```python
from build123d import *

# Parameters (mm, degrees)
SKETCH_1_W          = 5
SKETCH_1_H          = 20
SKETCH_1_H_2        = 5
SKETCH_1_W_2        = 20
EXTRUDE_1_DEPTH     = 20
CUT_EXTRUDE_1_REACH = 36.641
SKETCH_2_R          = 1.5
CUT_EXTRUDE_2_REACH = 39.749
SKETCH_3_R          = 1.5


with BuildPart() as part:
    # 草图1 → 凸台-拉伸1 (new body)
    with BuildSketch(Plane.XY):
        with Locations((2.5, -10)):
            Rectangle(SKETCH_1_W, SKETCH_1_H)
        with Locations((2.5, -22.5)):
            Rectangle(SKETCH_1_W, SKETCH_1_H_2)
        with Locations((-10, -22.5)):
            Rectangle(SKETCH_1_W_2, SKETCH_1_H_2)
    extrude(amount=EXTRUDE_1_DEPTH)

    # 草图2 → 切除-拉伸1 (cut, up to next)
    with BuildSketch(Plane(origin=(0, -20, 0), x_dir=(1, 0, 0), z_dir=(0, 1, 0)), mode=Mode.PRIVATE) as cut_extrude_1_sk1:
        with Locations(Location((-10, -10, 0), (0, 0, 180))):
            Circle(SKETCH_2_R)
    cut_extrude_1_tool1 = extrude(cut_extrude_1_sk1.sketch, amount=-CUT_EXTRUDE_1_REACH, mode=Mode.PRIVATE) & part.part
    add(cut_extrude_1_tool1.solids().sort_by_distance((-10, -20, 10))[0], mode=Mode.SUBTRACT)

    # 草图3 → 切除-拉伸2 (cut, up to next)
    with BuildSketch(Plane.ZY, mode=Mode.PRIVATE) as cut_extrude_2_sk1:
        with Locations(Location((10, -10, 0), (0, 0, 270))):
            Circle(SKETCH_3_R)
    cut_extrude_2_tool1 = extrude(cut_extrude_2_sk1.sketch, amount=-CUT_EXTRUDE_2_REACH, mode=Mode.PRIVATE) & part.part
    add(cut_extrude_2_tool1.solids().sort_by_distance((0, -10, 10))[0], mode=Mode.SUBTRACT)


solid = part.part
```
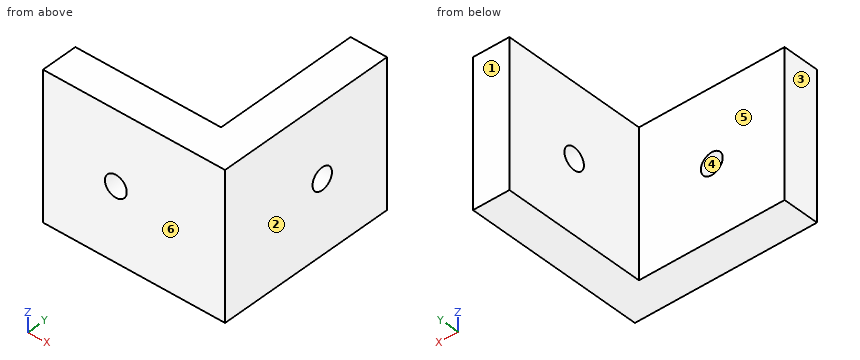
Input: part model. Units: mm. Frame: model coordinates. Face numbers are marked on the shaded views. A direction names the side the tool comes from. Give positions to 0.01 mm unless a question says otherwise; leave off trailing zeros. Order: outer loops, then holes, each group sorted by start corner. A loop starts at its lowest first (then second) coordinate and runs counter-clockwise, first axis right, second up. Notation, with made-up numbers: (-0.75, 61) -> (25.25, 61) arc R23 cw to (25.25, 98) -> close; hole circle Ø9 at (63.5, -4). An arc over 180 degrees is marked (long way). Write each question's results on one line, items separated by ' | '. Start each with the question number.
Item 1: Cut plane A-A on x = -10. Return the cut outline in (y, z), then the cut area to 3 significant figures.
Item 2: Mould query, pull axis X, two halves, no side actions, for the marked faces 1, 2, 3 and 4. Classes: pulls with the +X half, pulls with the -X half, needs draft (parallel to the pull), parting line crosses it, or undercut.
Item 3: Cut plane C-C on z = 9.25. Return the cut outline in (x, y), then the cut area to 3 significant figures.
Item 4: Contact query for flat-ended pins moving along their axis: P1, Ø4, axis at x = -12.5, z = 3.5, coming from the +Y side; P2, Ø2, axis at y = -7.5, z = 6, coming from the -X side; P3, Ø1.8, axis at y = -10, z = 10, coming from the +X side. Output: stop coordinate, or through.
Item 5: Line query: line 1 (Z direction, x = 1.25, y = -10); line 2 (X direction, y = -18.75, z = 4.5); line 3 (Y direction, x = -4.75, z = 16.5). Output: solid intervals per line, ascending.
Item 6: Set-up query: the marked faces 5 and 6. Return all of +Z, -Z, +X, -X, +Y, -Y with unobstructed straight access to the full face (end or side cutting, diameter ignored); none if empty.
Item 7: Cut plane D-D on z = 12. Return the cut outline in (x, y), then the cut area to 3 significant figures.
Item 8: Cut plane B-B on y = -10. Return the cut outline in (x, z).
Established:
1) outline: (-25, 0) -> (-20, 0) -> (-20, 8.5) -> (-25, 8.5) -> close; (-25, 11.5) -> (-20, 11.5) -> (-20, 20) -> (-25, 20) -> close | area: 85.0 mm^2
2) face 1: needs draft | face 2: pulls with the +X half | face 3: pulls with the -X half | face 4: undercut
3) outline: (-20, -25) -> (-11.3, -25) -> (-11.3, -20) -> (-20, -20) -> close; (-8.7, -25) -> (5, -25) -> (5, -11.3) -> (0, -11.3) -> (0, -20) -> (-8.7, -20) -> close; (0, -8.7) -> (5, -8.7) -> (5, 0) -> (0, 0) -> close | area: 199 mm^2
4) P1: y = -20 | P2: x = 0 | P3: through
5) line 1: 0 to 8.5, 11.5 to 20 | line 2: 0 to 5 | line 3: -25 to -20
6) face 5: +Z, -Z, -X, +Y | face 6: +Z, -Z, +X, -X, -Y
7) outline: (-20, -25) -> (5, -25) -> (5, 0) -> (0, 0) -> (0, -20) -> (-20, -20) -> close | area: 225 mm^2
8) outline: (0, 0) -> (5, 0) -> (5, 8.5) -> (0, 8.5) -> close; (0, 11.5) -> (5, 11.5) -> (5, 20) -> (0, 20) -> close
